Design review of the part built by this model. Coordinates are the model's own, in mm. A direction names the side the tool comes from. Coordinates: 2 decimals unless noted, no trailing zeros. Write each loop counter-clockwise with the first axis right and the second up, starting at its lowest first coordinate (ties: lowest second). Pieces come first, ordered by that corner, then holes. Notation, with made-up numbers: M -7,-28 L -1,-28 A20 ccw -1,1 Z; hole C -9,80.25 d8. An arc over 180 degrees is marked long. Write item = value, one per line.
```python
from build123d import *

# Parameters (mm, degrees)
F1_DEPTH      = 84.582
F3_START      = 3.048
F3_DEPTH      = 77.724
F5_DEPTH      = 87.63
F5_DEPTH_BACK = 5.08


with BuildPart() as f1:
    # F0 (on Top) → F1 (new body)
    with BuildSketch(Plane.XY):
        Polygon((17.4885243177, -16.4683610201), (34.9770486355, -16.4683610201), (37.0173789561, 24.9211471528), (33.228199929, 27.5444276631), (27.9816426337, 27.5444276631), (21.8606535345, 24.9211471528), (17.4885243177, 18.2172134519), align=None)
    extrude(amount=F1_DEPTH)

    # F2 (on Top) → F3 (join)
    with BuildSketch(Plane.XY.offset(F3_START)):
        Polygon((63.1398186088, 9.1814752668), (20.5844063312, 0), (22.9162164032, -15.0109836832), (65.4716193676, -4.809344653), (68.0949017406, 0), (68.0949017406, 6.2667215243), align=None)
        Polygon((59.933591634, 22.5893463939), (37.1985062957, 22.5893463939), (22.9162164032, 22.5893463939), (22.9162164032, 13.2621303201), (59.933591634, 13.2621303201), (63.1398186088, 18.508689478), align=None)
    extrude(amount=F3_DEPTH)

    # F4 (on Top) → F5 (join, two sides)
    with BuildSketch(Plane.XY) as f5_sk:
        Polygon((33.8941030204, 18.2172134519), (37.3918153346, 15.0109836832), (45.1184251433, 16.9914124986), (41.4724685252, 13.0139971915), (46.6038940806, 13.0139971915), (50.2498506988, 16.9914124986), (54.5888580382, 13.0139971915), (59.3584632455, 18.2172134519), (59.3584632455, 23.4637726098), (54.5888580382, 27.8359018266), (50.2498506988, 27.8359018266), (46.2420737325, 23.4637726098), (41.4724685252, 27.8359018266), (35.6429591775, 27.8359018266), (33.8941030204, 23.4637726098), align=None)
    extrude(amount=F5_DEPTH)
    extrude(f5_sk.sketch, amount=-F5_DEPTH_BACK)


solid = f1.part
```
Q1. Consider section C-C, the plane y = -9.5. State the section outline as (x, z) points.
Check result:
outline = M 17.49,0 L 35.32,0 L 35.32,3.05 L 45.9,3.05 L 45.9,80.77 L 35.32,80.77 L 35.32,84.58 L 17.49,84.58 Z
Q2. Wall thickness on line 1 (Z direction, x = 62, y = 17.5); line 2 (Y direction, x = 28, z = 32); line 3 (X direction, y = -15, z = 70): over which ranges is each line inside the solid? List them lowest first.
Check result:
line_1 = 3.05 to 80.77
line_2 = -16.47 to 27.54
line_3 = 17.49 to 35.05
Q3. Machinability: for faces 5 (the flat face through (31, 27.544, 42)), 6 (the flat face through (49.74, 6.29, 41.37)), 7 (the flat face through (61.514, 15.849, 41.366)), 8 (the flat face through (51, 14, 80.772)), 9 (the flat face through (51, -1, 80.772)), which of the approach directions +Z, -Z, +X, -X, +Y, -Y give a long, thin tool a straight path to every point of the face, cutting with its end or side? Answer none if there is none.
Check result:
face_5 = +Z, -Z, -X, +Y
face_6 = +Z, -Z
face_7 = +Z, -Z, +X
face_8 = +Z, -Y
face_9 = +Z, +X, -Y
Q4. Consider section B-B, the plane x = 38.5. State the section outline as (y, z) points, and give its area (3 significant figures).
Check result:
outline = M -11.28,3.05 L 3.87,3.05 L 3.87,80.77 L -11.28,80.77 Z; M 13.26,3.05 L 15.3,3.05 L 15.3,-5.08 L 27.84,-5.08 L 27.84,87.63 L 15.3,87.63 L 15.3,80.77 L 13.26,80.77 Z
area = 2,500 mm²
Q5. The part is to be moulded in two halves that separate along Y. For faces 1 (the flat face through (41, 15, 80.772)), 2 (the flat face through (33.894, 21, 86)), 3 (the flat face through (39, 27.836, 42)), 4 (the flat face through (26, -16.468, 42)), say which applies: +Y half, -Y half, draft (parallel to the pull), parting line (faces both ways), or undercut.
Check result:
face_1 = undercut
face_2 = draft
face_3 = +Y half
face_4 = -Y half
Q6. Consider section D-D, the plane x = 30. State the section outline as (y, z) points, and give its area (3 significant figures).
Check result:
outline = M -16.47,0 L 27.54,0 L 27.54,84.58 L -16.47,84.58 Z
area = 3,720 mm²
Q7. For P1, Ø3, axis at x = 27.5, y = 6.5, coming from the -Z side; P2, Ø10.5, axis at x = 58.5, y = 4, coming from the -Z side; P3, Ø2, axis at x = 48, z = 43, coming from the +Y side, all flat-tipped, find the tip position at first contact; note any pin that passes through.
Check result:
P1 = 0
P2 = 3.05
P3 = 26.47
